Work out the finished part from the listing and answer in its coordinate system (mm). Face numbers are marked on the shaded views. A direction names the side the tool comes from. Round coordinates to 2 decimals unless told otherwise and drop trailing zeros. Order: outer loops, then holes, each group sorted by start corner. A loop starts at its lowest first (then second) coordinate and runs counter-clockwise, first axis right, second up. Notation, with made-up numbers: (61, 43.5) - (102, 43.5) arc R26 cw to (102, 82.5) - close; hole circle Ø9 at (77.25, 80). An arc over 180 degrees is marked (long way). Use CSV: the item, a comma, the result in double quotes.
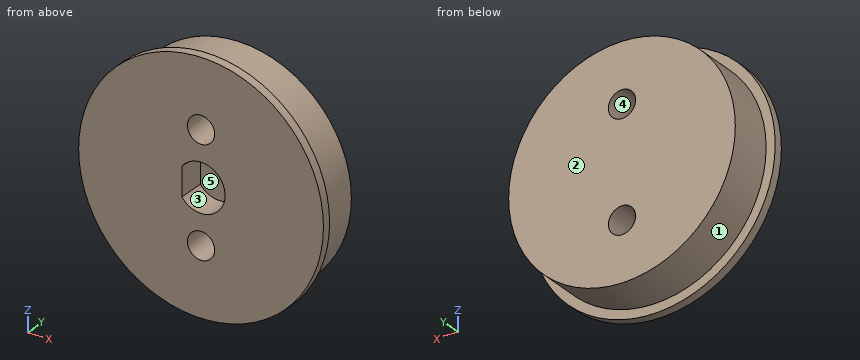
Autodesk Inventor part; units mm, degrees
ref_plane "YZ Plane" through (0, 0, 0) normal (1, 0, 0) x (0, 1, 0)
ref_plane "XZ Plane" through (0, 0, 0) normal (0, 1, 0) x (-1, 0, 0)
ref_plane "XY Plane" through (0, 0, 0) normal (0, 0, 1) x (1, 0, 0)
sketch "Szkic1" plane through (0, 0, 0) normal (0, 1, 0) x (-1, 0, 0)
  circle A0 centre (0, 0) radius 13.5
  dimension "d0" = 27
extrude "Wyciągnięcie proste1" add sketch "Szkic1" along normal blind 1
sketch "Szkic2" plane through (0, 1, 0) normal (0, 1, 0) x (1, 0, 0)
  circle A0 centre (0, 0) radius 12.5
  dimension "d3" = 25
extrude "Wyciągnięcie proste2" add sketch "Szkic2" along normal blind 5
sketch "Szkic3" plane through (0, 6, 0) normal (0, 1, 0) x (1, 0, 0)
  circle A0 centre (0, -6) radius 1.5
  point P0 (0, 0)
  dimension "d6" = 3
  dimension "d7" = 6
extrude "Wyciągnięcie proste3" cut sketch "Szkic3" against normal up to surface (6 mm away)
mirror "Odbij2" about plane through (0, 0, 0) normal (0, 0, 1) of "Wyciągnięcie proste3"
sketch "Sketch4" plane through (0, 0, 0) normal (0, -1, 0) x (1, 0, 0)
  arc A0 (-2.12, -1.59) -> (-2.12, 1.59) centre (0, 0) ccw
  line L0 (-2.12, 1.59) -> (-2.12, -1.59)
  dimension "d10" = 5.3
  dimension "d11" = 3.18
extrude "Extrusion4" cut sketch "Sketch4" against normal blind 3
properties part number "InputShaft3_3DPrint"
(1) Find section A-A (x = 0). Determine the outline of the cut face in (y, z).
Findings below:
outline,"(0, -13.5) - (1, -13.5) - (1, -12.5) - (6, -12.5) - (6, -7.5) - (0, -7.5) - close; (0, -4.5) - (6, -4.5) - (6, 4.5) - (0, 4.5) - (0, 2.65) - (3, 2.65) - (3, -2.65) - (0, -2.65) - close; (0, 7.5) - (6, 7.5) - (6, 12.5) - (1, 12.5) - (1, 13.5) - (0, 13.5) - close"
(2) Find section B-B (z = 5.25). Determine the outline of the cut face in (x, y), and give its area (3 significant figures).
Findings below:
outline,"(-12.44, 0) - (-1.3, 0) - (-1.3, 6) - (-11.34, 6) - (-11.34, 1) - (-12.44, 1) - close; (1.3, 0) - (12.44, 0) - (12.44, 1) - (11.34, 1) - (11.34, 6) - (1.3, 6) - close"
area,"123 mm²"
(3) Find the intervals of material crossed by L1, parallel to Z at x = 0, y = 3.3; L2, parallel to Z at x = 0, y = 1.5; L3, parallel to Z at x = -1, y = 1.2, in increasing order. Write a range as from..to.
Findings below:
L1,"z = -12.5..-7.5, -4.5..4.5, 7.5..12.5"
L2,"z = -12.5..-7.5, -4.5..-2.65, 2.65..4.5, 7.5..12.5"
L3,"z = -12.46..-7.12, -4.88..-2.45, 2.45..4.88, 7.12..12.46"
(4) Find section C-C (y = 4.7). Determine the outline of the cut face in (x, z), and give its area (3 significant figures).
Findings below:
outline,"circle Ø25 at (0, 0); hole circle Ø3 at (0, -6); hole circle Ø3 at (0, 6)"
area,"477 mm²"
(5) Find section D-D (z = 8.5). Determine the outline of the cut face in (x, y).
Findings below:
outline,"(-10.49, 0) - (10.49, 0) - (10.49, 1) - (9.17, 1) - (9.17, 6) - (-9.17, 6) - (-9.17, 1) - (-10.49, 1) - close"
(6) The mould has two halves that part along X. Classify the marked faces 1, 2 and 3: released by +X, released by -X, zero draft, split by the parting line, or undercut.
Findings below:
face 1,"split by the parting line"
face 2,"zero draft"
face 3,"undercut"
(7) Each of these flat-tipped pins is pushed along its axis until it touches: pin 1 (1 mm diameter, centred on y = 5.5, z = -4, fed in from +X); pin 2 (1.5 mm diameter, centred on x = 7, y = 3.5, fed in from +Z); pin 3 (4 mm diameter, centred on x = 0, z = 0, fed in from -Y); pin 4 (5 mm diameter, centred on x = -5, z = -1.5, fed in from -Y). Where does it stop, or does it pass through?
Findings below:
pin 1,"stops at x = 12"
pin 2,"stops at z = 10.83"
pin 3,"stops at y = 3"
pin 4,"stops at y = 0"
(8) For the marked faces 4 and 5, determine the directions among +Z, -Z, +X, -X, +Y, -Y from which every point of the face is accessible in a straight line to the end or side of a thin tool.
Findings below:
face 4,"+Y, -Y"
face 5,"-Y"
